Verification items for the finished model (mm, model axes). A direction names the side the tool comes from. Give positions to 0.01 mm unless a question says otherwise; leave off trailing zeros. Loops run counter-clockwise (first coordinate to the right, second up) from the corner with the lowest first, then second, coordinate; pieces in that order, holes last. Notation, with made-up numbers: (81.25, -9) -> (85.25, -9) arc R20 ccw to (85.25, 28) -> close; hole circle Ø8 at (7.25, 58). An arc over 180 degrees is marked (long way). Answer in a Markdown table with one row per item. Add a question column.
Q1. Gauge pin test, flat ends, axial feed: P1, Ø5.5, axis at x = 8, y = 21.5, coming from the +Z side; P2, Ø1.5, axis at x = 43, y = 21, coming from the -Z side; P3, Ø10, axis at x = 14.5, y = 27.5, coming from the +Z side; P4, Ø10, axis at y = 18, z = 60, coming from the -X side. Record the tip position at first contact, or that the pin passes through.
Q2. Section check B-B on x = 43.5. Enter the section's corners in (y, z), and give its area (3 significant figures).
Q3. Material ranges on probe 1 along Z at (x, y) = (28, 24.5); probe 2 along Z at (x, y) = (8.5, 19.5); probe 3 along X at (y, z) = (5.5, 104.5), recorded low to high.
Q4. Section check C-C on z = 102.5. Enter the section's corners in (x, y), and give its area (3 significant figures).
Q5. Set-up check for faces 1 (the face through (47, 0, 49)), 2 (the face through (9, 17, 6)), 3 (the face through (46, 16, -13)): record each of +Z, -Z, +X, -X, +Y, -Y from which the full face is reachable in a straight line by a thin tool's end or side.
Q6. Section check A-A on y = 19. Enter the section's corners in (x, z).
```python
from build123d import *

# Parameters (mm, degrees)
BOX002_W     = 48
BOX002_H     = 33.1
BOX002_DEPTH = 125
BOX001_W     = 11
BOX001_H     = 33.1
BOX001_DEPTH = 31
BOX_W        = 66
BOX_H        = 33.1
BOX_DEPTH    = 6
BOX003_W     = 10
BOX003_H     = 33.1
BOX003_DEPTH = 31


with BuildPart() as cubo002:
    # Box002 → Box002 (new body)
    with BuildSketch(Plane(origin=(18, 0, 0), x_dir=(1, 0, 0), z_dir=(0, 0, 1))):
        with Locations((24, 16.55)):
            Rectangle(BOX002_W, BOX002_H)
    extrude(amount=BOX002_DEPTH)


with BuildPart() as cubo001:
    # Box001 → Box001 (new body)
    with BuildSketch(Plane(origin=(46, 0, -25), x_dir=(1, 0, 0), z_dir=(0, 0, 1))):
        with Locations((5.5, 16.55)):
            Rectangle(BOX001_W, BOX001_H)
    extrude(amount=BOX001_DEPTH)


with BuildPart() as cubo:
    # Box → Box (new body)
    with BuildSketch(Plane.XY):
        with Locations((33, 16.55)):
            Rectangle(BOX_W, BOX_H)
    extrude(amount=BOX_DEPTH)


with BuildPart() as fusion:
    # Box003 → Box003 (new body)
    with BuildSketch(Plane(origin=(56, 0, -25), x_dir=(1, 0, 0), z_dir=(0, 0, 1))):
        with Locations((5, 16.55)):
            Rectangle(BOX003_W, BOX003_H)
    extrude(amount=BOX003_DEPTH)

    # Fusion: union Cubo002, Cubo001, Cubo
    add(cubo002.part)
    add(cubo001.part)
    add(cubo.part)


solid = fusion.part
```
Taken from the geometry:
| question | item | result |
|---|---|---|
| 1 | P1 | stops at z = 6 |
| 1 | P2 | stops at z = 0 |
| 1 | P3 | stops at z = 125 |
| 1 | P4 | stops at x = 18 |
| 2 | outline | (0, 0) -> (33.1, 0) -> (33.1, 125) -> (0, 125) -> close |
| 2 | area | 4,140 mm² |
| 3 | probe 1 | z = 0 to 125 |
| 3 | probe 2 | z = 0 to 6 |
| 3 | probe 3 | x = 18 to 66 |
| 4 | outline | (18, 0) -> (66, 0) -> (66, 33.1) -> (18, 33.1) -> close |
| 4 | area | 1,590 mm² |
| 5 | face 1 | +Z, -Z, +X, -X, -Y |
| 5 | face 2 | +Z, -X, +Y, -Y |
| 5 | face 3 | -Z, -X, +Y, -Y |
| 6 | outline | (0, 0) -> (46, 0) -> (46, -25) -> (66, -25) -> (66, 125) -> (18, 125) -> (18, 6) -> (0, 6) -> close |
